Verification items for the finished model (mm, model axes). Face numbers are marked on the shaded views. A direction names the side the tool comes from. Round coordinates to 2 decimals unless told otherwise and drop trailing zeros. Loops run counter-clockwise (first coordinate to the right, second up) from the corner with the lowest first, then second, coordinate; pieces in that order, holes last. Notation, with made-up numbers: M -8,-8.75 L 44,-8.75 A20 ccw 44,12.25 Z; hole C 84.5,-21.75 d4. An arc over 180 degrees is marked long. One line per item, written item: value.
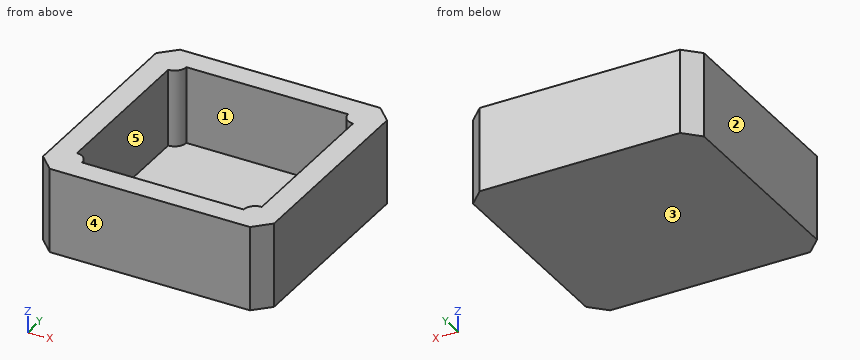
from build123d import *

# Parameters (mm, degrees)
F0_W     = 30
F0_H     = 30
F1_DEPTH = 1
F2_W     = 30
F2_H     = 30
F3_DEPTH = 10
F4_SIZE  = 2


with BuildPart() as f1:
    # F0 (on Top) → F1 (new body)
    with BuildSketch(Plane.XY):
        with Locations((15, 15)):
            Rectangle(F0_W, F0_H)
    extrude(amount=F1_DEPTH)

    # F2 (on face) → F3 (join)
    with BuildSketch(Plane.XY.offset(1)):
        with Locations((15, 15)):
            Rectangle(F2_W, F2_H)
        with BuildLine():
            Line((3, 4.5), (3, 25.5))
            ThreePointArc((3, 25.5), (4.06066, 25.93934), (4.5, 27))
            Line((4.5, 27), (25.5, 27))
            ThreePointArc((25.5, 27), (25.93934, 25.93934), (27, 25.5))
            Line((27, 25.5), (27, 4.5))
            ThreePointArc((27, 4.5), (25.93934, 4.06066), (25.5, 3))
            Line((25.5, 3), (4.5, 3))
            ThreePointArc((4.5, 3), (4.06066, 4.06066), (3, 4.5))
        make_face(mode=Mode.SUBTRACT)
    extrude(amount=F3_DEPTH)

    # F4
    f4_edges = [f1.edges().sort_by_distance(p)[0] for p in [
        (30, 30, 5.5),
        (30, 0, 5.5),
        (0, 0, 5.5),
        (0, 30, 5.5),
    ]]
    chamfer(f4_edges, length=F4_SIZE)


solid = f1.part
(1) Sectioned sample at B-B on y = 15.5. Enter the section's corners in (x, z).
Completed:
outline: M 0,0 L 30,0 L 30,11 L 27,11 L 27,1 L 3,1 L 3,11 L 0,11 Z
(2) Thickness scan on L1, parallel to X at y = 17.75, z = 3; L2, parallel to Z at x = 19.5, y = 8. Record the ranges inside material, lowest first. Write a range as from..to.
Completed:
L1: x = 0..3, 27..30
L2: z = 0..1
(3) Depth check by flat-ended pin: pin 1 Ø6 at (x, y) = (22, 19) entering from +Z. Enter the tip coordinate at first touch or a pass-through.
Completed:
pin 1: stops at z = 1
(4) Mould release check, pull along Y, two halves, no side actions. Record for the marked faces 3, 4 and 5: +Y half, -Y half, draft (parallel to the pull), parting line (faces both ways), or undercut.
Completed:
face 3: draft
face 4: -Y half
face 5: undercut
(5) Tool access check on the marked faces 1 and 2. Record the directions out of +Z, -Z, +X, -X, +Y, -Y that give a thin tool (end or side, any length) a straight path to the whole face; none if there is none.
Completed:
face 1: +Z
face 2: +Z, -Z, -X, +Y, -Y
(6) Sectioned sample at A-A on z = 5.75. Enter the section's corners in (x, y).
Completed:
outline: M 0,2 L 2,0 L 28,0 L 30,2 L 30,28 L 28,30 L 2,30 L 0,28 Z; hole M 3,4.5 A1.5 cw 4.5,3 L 25.5,3 A1.5 cw 27,4.5 L 27,25.5 A1.5 cw 25.5,27 L 4.5,27 A1.5 cw 3,25.5 Z
